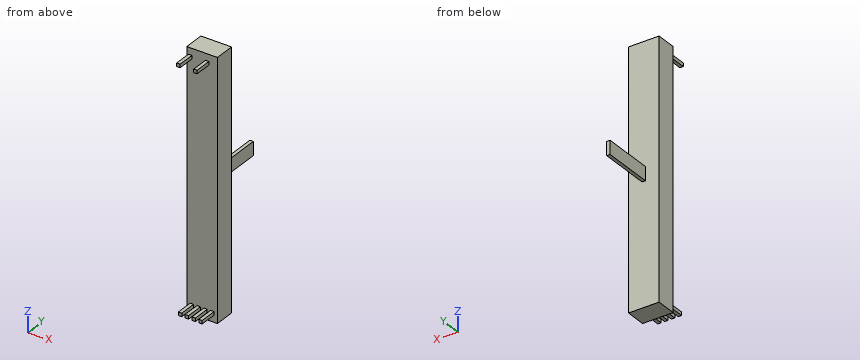
from build123d import *

# Parameters (mm, degrees)
SKETCH1_W           = 9
SKETCH1_H           = 75
BOSS_EXTRUDE1_DEPTH = 6
SKETCH2_W           = 1
SKETCH2_H           = 4
BOSS_EXTRUDE2_DEPTH = 15
SKETCH4_W           = 1
SKETCH4_H           = 1
BOSS_EXTRUDE3_DEPTH = 5


with BuildPart() as part:
    # Sketch1 → Boss-Extrude1 (new body)
    with BuildSketch(Plane(origin=(0, 0, 0), x_dir=(1, 0, 0), z_dir=(0, 1, 0))):
        Rectangle(SKETCH1_W, SKETCH1_H)
    extrude(amount=BOSS_EXTRUDE1_DEPTH)

    # Sketch2 → Boss-Extrude2 (add)
    with BuildSketch(Plane(origin=(0, 6, 0), x_dir=(1, 0, 0), z_dir=(0, 1, 0))):
        with Locations((0, -0.071668646)):
            Rectangle(SKETCH2_W, SKETCH2_H)
    extrude(amount=BOSS_EXTRUDE2_DEPTH)

    # Sketch4 → Boss-Extrude3 (add)
    with BuildSketch(Plane.XZ):
        with Locations((-3.5, 35)):
            Rectangle(SKETCH4_W, SKETCH4_H)
        with Locations((1.5, 35)):
            Rectangle(SKETCH4_W, SKETCH4_H)
        with Locations((-3, -35)):
            Rectangle(SKETCH4_W, SKETCH4_H)
        with Locations((-1, -35)):
            Rectangle(SKETCH4_W, SKETCH4_H)
        with Locations((1, -35)):
            Rectangle(SKETCH4_W, SKETCH4_H)
        with Locations((3, -35)):
            Rectangle(SKETCH4_W, SKETCH4_H)
    extrude(amount=BOSS_EXTRUDE3_DEPTH)


solid = part.part
Geometry check sheet. Reference: the model listing, model coordinates, mm. Give positions to 0.01 mm unless a question says otherwise; leave off trailing zeros. Write each loop counter-clockwise with the first axis right and the second up, starting at its lowest first coordinate (ties: lowest second). Pieces come first, ordered by that corner, then holes. Notation, with made-up numbers: (32, 85) - (54, 85) arc R6 ccw to (54, 94) - close; hole circle Ø5 at (6, 58.5). An arc over 180 degrees is marked (long way). Put each result on its own line as item: value.
1. Go/stop test with flat-tipped pins: pin 1 (1.1 mm diameter, centred on y = -1.5, z = -35, fed in from -X); pin 2 (0.5 mm diameter, centred on y = -3, z = -35, fed in from +X); pin 3 (0.8 mm diameter, centred on x = 3, y = -3.5, fed in from -Z); pin 4 (4 mm diameter, centred on x = -1.5, z = -3.5, fed in from +Y). Record where each tip stops, or that it passes through.
Ans:
pin 1: stops at x = -3.5
pin 2: stops at x = 3.5
pin 3: stops at z = -35.5
pin 4: stops at y = 21
2. Sectioned sample at A-A, the plane y = 9.75. Enter the section's corners in (x, z).
Ans:
outline: (-0.5, -1.93) - (0.5, -1.93) - (0.5, 2.07) - (-0.5, 2.07) - close
3. Thickness scan on line 1 (Z direction, x = -0.25, y = 11); line 2 (Y direction, x = -2.75, z = -16); line 3 (Z direction, x = 1.75, y = -2). Record the ranges inside material, lowest first.
Ans:
line 1: z = -1.93 to 2.07
line 2: y = 0 to 6
line 3: z = 34.5 to 35.5
4. Sectioned sample at B-B, the plane z = -6.5. Enter the section's corners in (x, y).
Ans:
outline: (-4.5, 0) - (4.5, 0) - (4.5, 6) - (-4.5, 6) - close
